Part model, mm, in its own coordinate system. A direction names the side the tool comes from. Round coordinates to 2 decimals unless told otherwise and drop trailing zeros. Loops run counter-clockwise (first coordinate to the right, second up) from the corner with the lowest first, then second, coordinate; pieces in that order, holes last. Notation, with made-up numbers: M -14.5,45 L 13.5,45 A14 cw 13.5,49 Z; hole C 30,1.25 d4. An arc over 180 degrees is marked long. Write each question's results on one line, items separated by ' | '.
from build123d import *

# Parameters (mm, degrees)
EXTRUDE_1_DEPTH = 1
EXTRUDE_2_DEPTH = 18


with BuildPart() as part:
    # 草图1 → 凸台-拉伸1 (new body)
    with BuildSketch(Plane.XY):
        with BuildLine():
            Line((-3.132848788, 7.321546969), (5.667151212, 7.321546969))
            ThreePointArc((5.667151212, 7.321546969), (6.374257994, 7.02865375), (6.667151212, 6.321546969))
            Line((6.667151212, 6.321546969), (6.667151212, -1.478453031))
            ThreePointArc((6.667151212, -1.478453031), (6.374257994, -2.185559812), (5.667151212, -2.478453031))
            Line((5.667151212, -2.478453031), (-3.132848788, -2.478453031))
            ThreePointArc((-3.132848788, -2.478453031), (-3.839955569, -2.185559812), (-4.132848788, -1.478453031))
            Line((-4.132848788, -1.478453031), (-4.132848788, 6.321546969))
            ThreePointArc((-4.132848788, 6.321546969), (-3.839955569, 7.02865375), (-3.132848788, 7.321546969))
        make_face()
    extrude(amount=EXTRUDE_1_DEPTH)

    # 草图2 → 凸台-拉伸2 (add)
    with BuildSketch(Plane(origin=(0, 0, 0), x_dir=(-1, 0, 0), z_dir=(0, 0, -1))):
        with BuildLine():
            Line((-3.667151212, 5.121546969), (1.132848788, 5.121546969))
            ThreePointArc((1.132848788, 5.121546969), (1.698534213, 4.887232394), (1.932848788, 4.321546969))
            Line((1.932848788, 4.321546969), (1.932848788, 0.521546969))
            ThreePointArc((1.932848788, 0.521546969), (1.698534213, -0.044138456), (1.132848788, -0.278453031))
            Line((1.132848788, -0.278453031), (-3.667151212, -0.278453031))
            ThreePointArc((-3.667151212, -0.278453031), (-4.232836637, -0.044138456), (-4.467151212, 0.521546969))
            Line((-4.467151212, 0.521546969), (-4.467151212, 4.321546969))
            ThreePointArc((-4.467151212, 4.321546969), (-4.232836637, 4.887232394), (-3.667151212, 5.121546969))
        make_face()
    extrude(amount=EXTRUDE_2_DEPTH)


solid = part.part
Item 1: Band-saw the part on A-A on x = 0.5. Give the cut face in (y, z).
Filled sheet:
outline: M -2.48,0 L -0.28,0 L -0.28,-18 L 5.12,-18 L 5.12,0 L 7.32,0 L 7.32,1 L -2.48,1 Z
Item 2: Which spindle directions (+Z, -Z, +X, -X, +Y, -Y) get a long thin tool onto all of the face, cutting with end or side? Do faces 1 (the flat face through (1, -1, 0)), 2 (the flat face through (1, 5.122, -9)), 3 (the flat face through (-1.933, 2, -9)), 4 (the cylindrical face through (4.24, 4.88, -8.87)), 5 (the cylindrical face through (4.227, -0.05, -8.874)). Say none if no direction does.
Filled sheet:
face 1: -Z | face 2: -Z, +X, -X, +Y | face 3: -Z, -X, +Y, -Y | face 4: -Z, +X, +Y | face 5: -Z, +X, -Y
Item 3: Band-saw the part on C-C on x = 5.25. Give the cut face in (y, z), and give its area (3 significant figures).
Filled sheet:
outline: M -2.48,0 L 7.32,0 L 7.32,1 L -2.48,1 Z | area: 9.80 mm^2
Item 4: Drop flat-ended pins along their axis: P1, Ø1.1, axis at y = 2, z = -7, coming from the -X side; P2, Ø4, axis at x = 0.5, z = -4.5, coming from the +Y side; P3, Ø4, axis at y = 0, z = -4, coming from the +X side. Give the stop position or say it passes through.
Filled sheet:
P1: x = -1.93 | P2: y = 5.12 | P3: x = 4.47
Item 5: Band-saw the part on B-B on y = 2.5. Give the cut face in (x, z), and give its area (3 significant figures).
Filled sheet:
outline: M -4.13,0 L -1.93,0 L -1.93,-18 L 4.47,-18 L 4.47,0 L 6.67,0 L 6.67,1 L -4.13,1 Z | area: 126 mm^2
Item 6: Wall check: L1, parallel to Z at x = 6, y = 1.25; L2, parallel to Y at x = -1, z = -5.75; L3, parallel to X at y = 2, z = -15.75. Give the ranges that are in metal, low to high.
Filled sheet:
L1: 0 to 1 | L2: -0.28 to 5.12 | L3: -1.93 to 4.47
